Design review of the part shown in the three views and the two pictorial views. Dimensions are in mm from the part's minimum x, y and z. A direction names the side the tool comes from. Give positions to 0.01 mm unless a question says otherwise; leave off trailing zeros. Order: outer loops, then holes, each group sorted by start corner. A loop starts at its lowest first (then second) coordinate and runs counter-clockwise, first axis right, second up. Notation, with made-up numbers: (85, 63) - (102, 63) arc R15 cw to (102, 73) - close; hole circle Ø6 at (-29, -15). An arc over 180 degrees is marked (long way). Put each result on its own line as item: value. Start each with the question number.
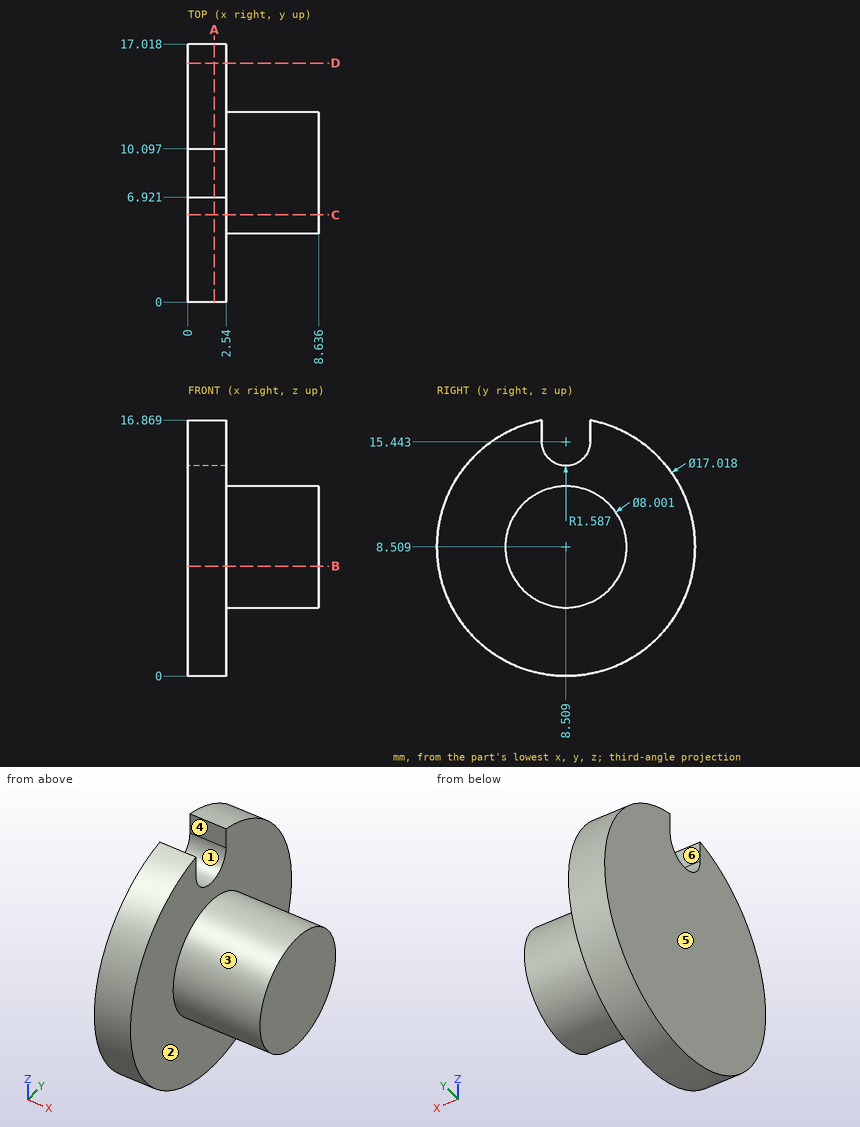
1. Add section C-C, the plane y = 5.75. Give the boundary of the cut face in (x, z) (1 decimal).
2. Wall thickness on line 1 (X direction, y = 1, z = 7.25); line 2 (Y direction, x = 1.25, z = 15.25) (1 decimal); line 3 (Z direction, x = 6.5, y = 8): over which ranges is each line inside the solid? List them lowest first. Write a range as from..to.
3. The part is to be moulded in two halves that separate along Y. For the marked faces 1, 2, 3 and 4, say which applies: released by +Y, released by -Y, zero draft, split by the parting line, or undercut.
4. Add section D-D, the plane y = 15.75. Give the boundary of the cut face in (x, z), then the cut area to 3 significant figures.
5. Clearance check with flat-ended pins moving along their axes: pin 1 (4 mm diameter, centred on x = 1.5, y = 3, fed in from +Z); pin 2 (6 mm diameter, centred on y = 12.5, z = 1.5, fed in from +X); pin 3 (1.1 mm diameter, centred on x = 1.5, z = 16, fed in from -Y) (1 decimal); pin 4 (3 mm diameter, centred on x = 5.5, y = 2.5, fed in from -Z). State where each tip first meets the part, or that it passes through.
6. Tool access review of the marked faces 5 and 6: name each direction out of +Z, -Z, +X, -X, +Y, -Y from which nothing blocks a thin tool from reaching the whole face with its end or side.
7. Add section A-A, the plane x = 1.75. Give the boundary of the cut face in (y, z) (1 decimal), then the cut area to 3 significant figures.
8. Add section B-B, the plane z = 7.25. Give the boundary of the cut face in (x, y) (1 decimal).
Found:
1. outline: (0, 0.5) - (2.5, 0.5) - (2.5, 5.6) - (8.6, 5.6) - (8.6, 11.4) - (2.5, 11.4) - (2.5, 16.6) - (0, 16.6) - close
2. line 1: x = 0..2.54
2. line 2: y = 3.3..6.9, 10.1..13.7
2. line 3: z = 4.54..12.48
3. face 1: undercut
3. face 2: zero draft
3. face 3: split by the parting line
3. face 4: undercut
4. outline: (0, 4.04) - (2.54, 4.04) - (2.54, 12.98) - (0, 12.98) - close
4. area: 22.7 mm^2
5. pin 1: stops at z = 16.26
5. pin 2: stops at x = 2.54
5. pin 3: stops at y = 3.6
5. pin 4: passes through
6. face 5: +Z, -Z, -X, +Y, -Y
6. face 6: +Z, +X, -X
7. outline: (6.9, 15.4) - (6.9, 16.9) arc R8.5 ccw (long way) to (10.1, 16.9) - (10.1, 15.4) arc R1.6 cw to start
7. area: 219 mm^2
8. outline: (0, 0.1) - (2.5, 0.1) - (2.5, 4.7) - (8.6, 4.7) - (8.6, 12.3) - (2.5, 12.3) - (2.5, 16.9) - (0, 16.9) - close
